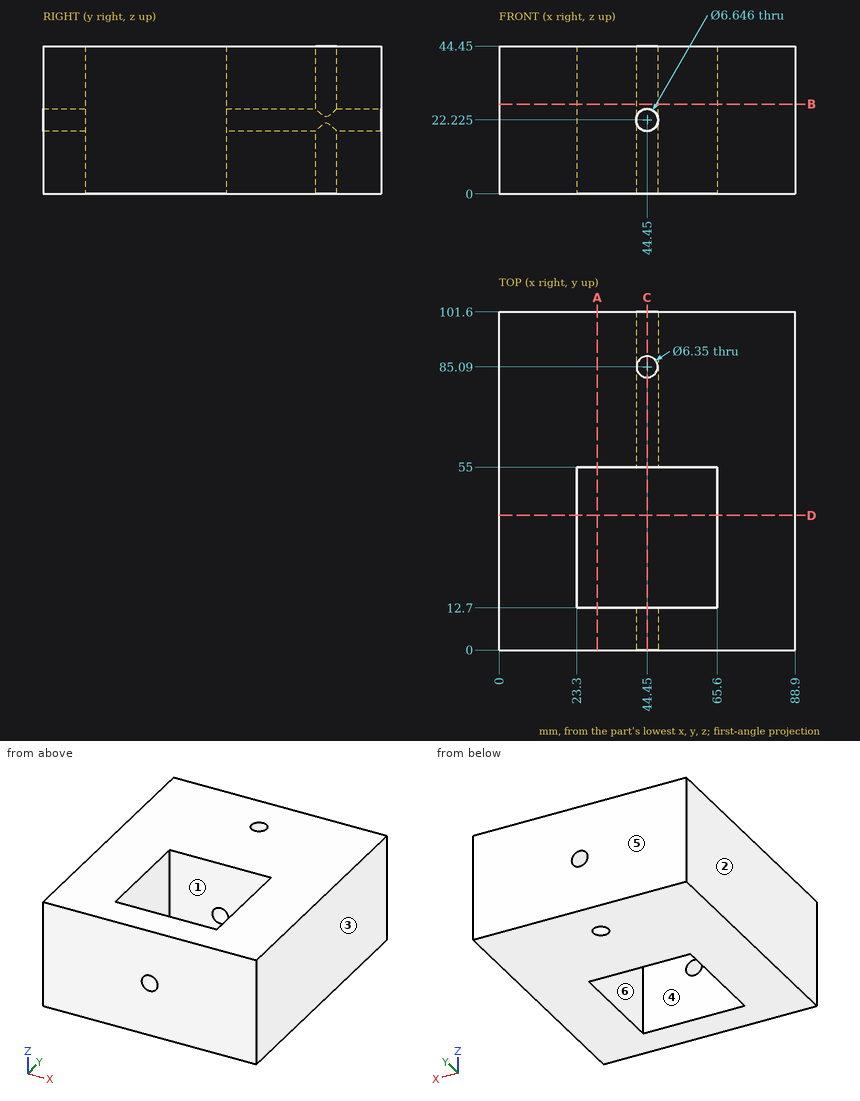
Job drawing, mm, ordinate dimensions from the low corner. One solid piece. A direction names the side the tool comes from. Give positions to 0.01 mm unless a question says otherwise; leave off trailing zeros. Loops run counter-clockwise (first coordinate to the right, second up) from the corner with the lowest first, then second, coordinate; pieces in that order, holes last. Notation, with made-up numbers: (13, 65.25) -> (36, 65.25) arc R21 ccw to (36, 71.25) -> close; hole circle Ø9 at (46.5, -15.5). An arc over 180 degrees is marked (long way). Write each question's results on one line, items separated by ' | '.
(1) Cut at D-D on y = 40.5. List the corners of the cut face in (x, z), and give its area (3 significant figures).
Geometry results:
outline: (0, 0) -> (23.3, 0) -> (23.3, 44.45) -> (0, 44.45) -> close; (65.6, 0) -> (88.9, 0) -> (88.9, 44.45) -> (65.6, 44.45) -> close | area: 2,070 mm²
(2) Cut at C-C on x = 44.45. Give the number of separate pieces and of enclosed holes in the cut face, and give its area (3 significant figures).
Geometry results:
separate pieces: 6 | enclosed holes: 0 | area: 2,000 mm²
(3) Cut at B-B on z = 27. List the corners of the cut face in (x, y) (3 decimals), and give its area (3 significant figures).
Geometry results:
outline: (0, 0) -> (88.9, 0) -> (88.9, 101.6) -> (0, 101.6) -> close; hole (23.3, 12.7) -> (65.6, 12.7) -> (65.6, 55) -> (23.3, 55) -> close; hole circle Ø6.35 at (44.45, 85.09) | area: 7,210 mm²
(4) Cut at A-A on x = 29.5. List the corners of the cut face in (y, z).
Geometry results:
outline: (0, 0) -> (12.7, 0) -> (12.7, 44.45) -> (0, 44.45) -> close; (55, 0) -> (101.6, 0) -> (101.6, 44.45) -> (55, 44.45) -> close
(5) Tool access for the marked faces 1 and 2: list every direction of +Z, -Z, +X, -X, +Y, -Y with a clear straight run to the whole face (end or side of a thin tool).
Geometry results:
face 1: +Z, -Z | face 2: +Z, -Z, -X, +Y, -Y
(6) Probe line 1 along Y through (x, z) = (44.45, 16.25) (3 decimals); line 2 along Y through (x, z) = (25, 8); line 3 along Z through (x, y) = (44.45, 3.5). List the from-to ranges inside material, lowest first.
Geometry results:
line 1: y = 0 to 12.7, 55 to 81.915, 88.265 to 101.6 | line 2: y = 0 to 12.7, 55 to 101.6 | line 3: z = 0 to 18.9, 25.55 to 44.45
(7) Pull direction X, two halves, no side cores. Call the marked faces 3, 4, 5 and 6: released by +X, released by -X, zero draft, split by the parting line, or undercut.
Geometry results:
face 3: released by +X | face 4: undercut | face 5: zero draft | face 6: undercut
